Study the drawing (mm; zero at the part's minimum x, y, z) and answer. A direction names the side the tool comes from. Round coordinates to 2 decimals unless told otherwise and drop trailing zeros. Order: outer loops, then holes, each group sorted by start corner. A loop starts at its lowest first (then second) coordinate and runs counter-clockwise, first axis right, second up. Notation, with made-up numbers: M 14.25,-3.75 L 55.25,-3.75 A25 ccw 55.25,12.25 Z; hole C 34,-38.75 d6. An arc over 180 degrees is marked long. Put each result on its own line as item: value. Start each with the question number.
1. Each of these flat-tipped pins is pushed along its axis until it touches: pin 1 Ø6.5 at (x, y) = (10, 12.5) entering from +Z; pin 2 Ø1 at (y, z) = (13, 44) entering from -X; pin 3 Ø8 at (y, z) = (17, 24.5) entering from -X; pin 4 Ø10 at (y, z) = (16.5, 38) entering from +X. Where does it stop, or does it pass through?
2. The part is cut by section C-C (z = 37). Give the vertices of the cut face in (x, y), then the cut area to 3 significant figures.
3. Consider line 1 (Z direction, x = 16.75, y = 8.75); line 2 (Y direction, x = 11, z = 9.5). Determine where each line is inside the solid, lowest interval first.
4. The part is cut by section D-D (y = 7). Give the vertices of the cut face in (x, z).
5. Which of the six approach directions +Z, -Z, +X, -X, +Y, -Y give full straight-line access (tool end or side, diameter ignored) to the marked faces 1 and 2?
6. The part is cut by section A-A (y = 11). Give the vertices of the cut face in (x, z).
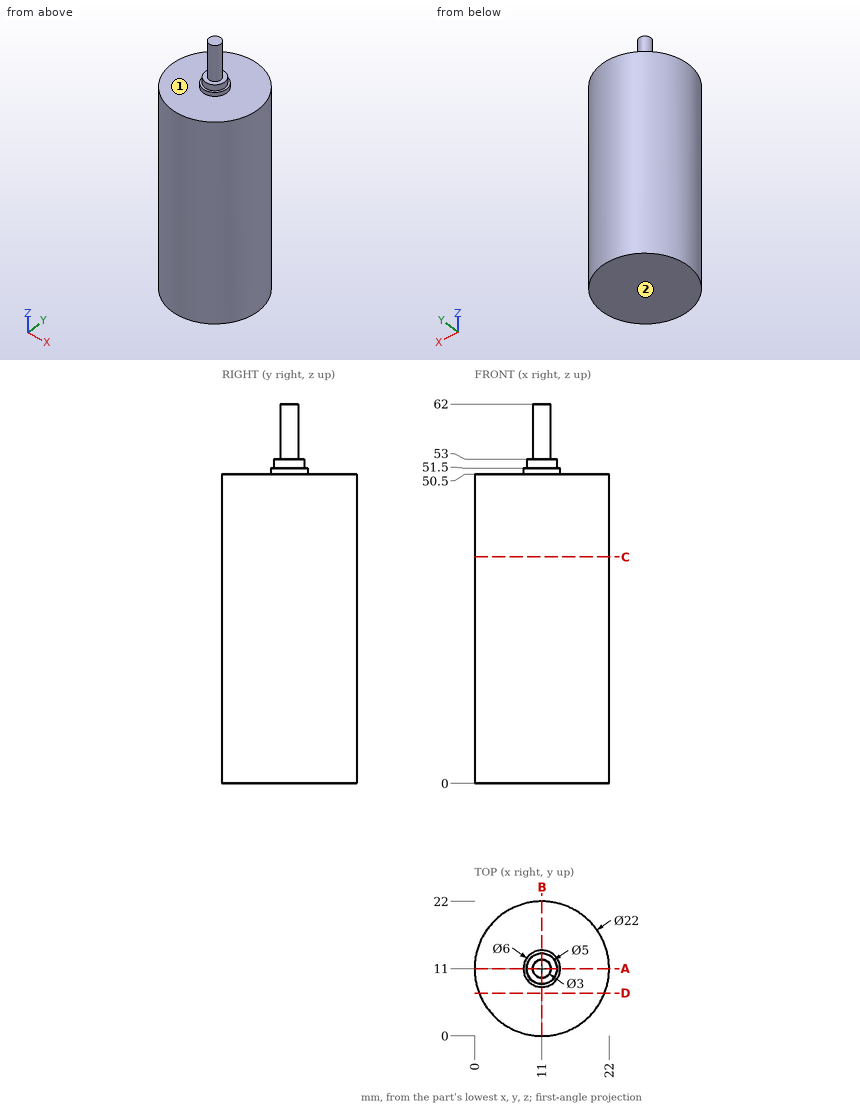
Resolved:
1. pin 1: z = 62
1. pin 2: x = 0.1
1. pin 3: x = 0.18
1. pin 4: x = 21.99
2. outline: C 11,11 d22
2. area: 380 mm2
3. line 1: 0 to 50.5
3. line 2: 0 to 22
4. outline: M 0.75,0 L 21.25,0 L 21.25,50.5 L 0.75,50.5 Z
5. face 1: +Z
5. face 2: -Z, +X, -X, +Y, -Y
6. outline: M 0,0 L 22,0 L 22,50.5 L 14,50.5 L 14,51.5 L 13.5,51.5 L 13.5,53 L 12.5,53 L 12.5,62 L 9.5,62 L 9.5,53 L 8.5,53 L 8.5,51.5 L 8,51.5 L 8,50.5 L 0,50.5 Z
